```python
from build123d import *

# Parameters (mm, degrees)
F1_DEPTH = 19.05
F2_R     = 6.35
F2_R_2   = 3.175
F3_DEPTH = 38.101


with BuildPart() as f1:
    # F0 (on Front) → F1 (new body, symmetric)
    with BuildSketch(Plane.XZ):
        Polygon((38.1, 19.05), (0, 19.05), (0, -19.05), (38.1, -19.05), (38.1, -6.35), (88.9, -6.35), (88.9, 6.35), (38.1, 6.35), align=None)
    extrude(amount=F1_DEPTH, both=True)

    # F2 (on face) → F3 (cut, through all)
    with BuildSketch(Plane.XY.offset(19.05)):
        with Locations((19.05, 0)):
            Circle(F2_R)
        with Locations((50.8, 6.35)):
            Circle(F2_R_2)
        with Locations((50.8, -6.35)):
            Circle(F2_R_2)
        with Locations((69.85, -6.35)):
            Circle(F2_R_2)
        with Locations((69.85, 6.35)):
            Circle(F2_R_2)
    extrude(amount=-F3_DEPTH, mode=Mode.SUBTRACT)


solid = f1.part
```
The listing builds one solid part. Answer for the finished solid, in the listing's coordinates (mm). A direction names the side the tool comes from. Coordinates: 2 decimals unless noted, no trailing zeros. Loops run counter-clockwise (first coordinate to the right, second up) from the corner with the lowest first, then second, coordinate; pieces in that order, holes last. Notation, with made-up numbers: (-31.75, 46) - (20.25, 46) arc R9 ccw to (20.25, 55) - close; hole circle Ø7 at (-19, -33). An arc over 180 degrees is marked (long way). Use a Markdown table: item, result. Add a question column.
1) The part is cut by section B-B, the plane x = 19.05. Give the vertices of the cut face in (y, z), and give its area (3 significant figures).
2) For faces 1 (the flat face through (38.1, 0, -13)), 2 (the flat face through (64, 0, 6.35)), 3 (the flat face through (0, 0, 0)), determine the directions among +Z, -Z, +X, -X, +Y, -Y from which every point of the face is accessible in a straight line to the end or side of a thin tool.
3) The part is cut by section A-A, the plane y = 0. Give the vertices of the cut face in (x, z), and give its area (3 significant figures).
4) Given pin 1 (14 mm diameter, centred on y = -4.5, z = 9.5, fed in from +X); pin 2 (1.5 mm diameter, centred on y = -1.5, z = 9.5, fed in from +X); pin 3 (11.5 mm diameter, centred on x = 58.5, y = -7.5, fed in from +Z); pin 4 (1.5 mm diameter, centred on x = 64, y = -15, fed in from -Z), each flat-ended and moving along its own axis, determine where each tip first touches the part or whether it passes through.
5) The part is cut by section D-D, the plane z = -13. Give the vertices of the cut face in (x, y).
6) Find the intervals of material crossed by line 1 (Y direction, x = 50.8, z = 1) (3 decimals); line 2 (Y direction, x = 50, z = 0); line 3 (Z direction, x = 67.5, y = -11), in increasing order.
7) The part is cut by section C-C, the plane x = 50.8. Give the vertices of the cut face in (y, z) (3 decimals).
Here are the results:
| question | item | result |
|---|---|---|
| 1 | outline | (-19.05, -19.05) - (-6.35, -19.05) - (-6.35, 19.05) - (-19.05, 19.05) - close; (6.35, -19.05) - (19.05, -19.05) - (19.05, 19.05) - (6.35, 19.05) - close |
| 1 | area | 968 mm^2 |
| 2 | face 1 | -Z, +X, +Y, -Y |
| 2 | face 2 | +Z, +X, +Y, -Y |
| 2 | face 3 | +Z, -Z, -X, +Y, -Y |
| 3 | outline | (0, -19.05) - (12.7, -19.05) - (12.7, 19.05) - (0, 19.05) - close; (25.4, -19.05) - (38.1, -19.05) - (38.1, -6.35) - (88.9, -6.35) - (88.9, 6.35) - (38.1, 6.35) - (38.1, 19.05) - (25.4, 19.05) - close |
| 3 | area | 1,610 mm^2 |
| 4 | pin 1 | stops at x = 88.9 |
| 4 | pin 2 | stops at x = 38.1 |
| 4 | pin 3 | stops at z = 6.35 |
| 4 | pin 4 | stops at z = -6.35 |
| 5 | outline | (0, -19.05) - (38.1, -19.05) - (38.1, 19.05) - (0, 19.05) - close; hole circle Ø12.7 at (19.05, 0) |
| 6 | line 1 | y = -19.05 to -9.525, -3.175 to 3.175, 9.525 to 19.05 |
| 6 | line 2 | y = -19.05 to -9.42, -3.28 to 3.28, 9.42 to 19.05 |
| 6 | line 3 | z = -6.35 to 6.35 |
| 7 | outline | (-19.05, -6.35) - (-9.525, -6.35) - (-9.525, 6.35) - (-19.05, 6.35) - close; (-3.175, -6.35) - (3.175, -6.35) - (3.175, 6.35) - (-3.175, 6.35) - close; (9.525, -6.35) - (19.05, -6.35) - (19.05, 6.35) - (9.525, 6.35) - close |
